Autodesk Fusion 360 part; units mm, degrees
sketch "Sketch1" plane through (0, 0, 0) normal (0, 1, 0) x (1, 0, 0)
  line L0 (2, -3.5) -> (30.5, -3.5)
  line L1 (30.5, -3.5) -> (30.5, -2)
  line L2 (30.5, -2) -> (2, -2)
  line L3 (2, -2) -> (2, -3.5)
  line L4 (12.5, -3.5) -> (20, -3.5)
  line L5 (20, -3.5) -> (20, -6.5)
  line L6 (20, -6.5) -> (12.5, -6.5)
  line L7 (12.5, -6.5) -> (12.5, -3.5)
  line L8 (12.1, -6.9) -> (20.4, -6.9)
  line L9 (20.4, -6.9) -> (20.4, -3.1)
  line L10 (20.4, -3.1) -> (12.1, -3.1)
  line L11 (12.1, -3.1) -> (12.1, -6.9)
  line L12 (0, -8.9) -> (32.5, -8.9)
  line L13 (32.5, -8.9) -> (32.5, 0)
  line L14 (32.5, 0) -> (0, 0)
  line L15 (0, 0) -> (0, -8.9)
  line L16 (30.5, -3.7) -> (26.5, -3.7)
  line L17 (26.5, -3.7) -> (26.5, -4.7)
  line L18 (26.5, -4.7) -> (30.5, -4.7)
  line L19 (30.5, -4.7) -> (30.5, -3.7)
  line L20 (26.5, -1.8) -> (30.5, -1.8)
  line L21 (30.5, -1.8) -> (30.5, -0.8)
  line L22 (30.5, -0.8) -> (26.5, -0.8)
  line L23 (26.5, -0.8) -> (26.5, -1.8)
  line L24 (2, -4.7) -> (6, -4.7)
  line L25 (6, -4.7) -> (6, -3.7)
  line L26 (6, -3.7) -> (2, -3.7)
  line L27 (2, -3.7) -> (2, -4.7)
  line L28 (2, -1.8) -> (6, -1.8)
  line L29 (6, -1.8) -> (6, -0.8)
  line L30 (6, -0.8) -> (2, -0.8)
  line L31 (2, -0.8) -> (2, -1.8)
  dimension "d1" = 28.5
  dimension "d2" = 1.5
  dimension "d3" = 7.5
  dimension "d4" = 3
  dimension "d5" = 10.5
  dimension "d6" = 0.4
  dimension "d7" = 0.4
  dimension "d8" = 0.4
  dimension "d9" = 0.4
  dimension "d10" = 2
  dimension "d11" = 2
  dimension "d12" = 2
  dimension "d13" = 2
  dimension "d30" = 4
  dimension "d31" = 1
  dimension "d32" = 0.2
  dimension "d33" = 4
  dimension "d34" = 4
  dimension "d35" = 1
  dimension "d36" = 0.2
  dimension "d37" = 4
  dimension "d38" = 4
  dimension "d39" = 1
  dimension "d40" = 4
  dimension "d41" = 1
  dimension "d42" = 4
  dimension "d43" = 4
  dimension "d44" = 0.2
  dimension "d45" = 0.2
extrude "Extrude1" add sketch "Sketch1" along normal blind 2 contours L0 L1 L2 L3 L9 L10 L11 | L12 L13 L14 L15 | L16 L17 L18 L19 | L20 L21 L22 L23 | L24 L25 L26 L27 | L28 L29 L30 L31
extrude "Extrude4" cut 1 faces at (28.4667, 2, 4) along direction (0, -1, 0) blind 1
extrude "Extrude5" add sketch "Sketch1" against normal blind 4 contours L16 L17 L18 L19 | L20 L21 L22 L23 | L24 L25 L26 L27 | L28 L29 L30 L31
sketch "Sketch3" plane through (0, 0, 4.7) normal (0, 0, 1) x (-1, 0, 0)
  line L0 (-6, 0) -> (-2, 0)
  line L1 (-2, 0) -> (-2, 4)
  line L2 (-2, 4) -> (-6, 4)
  line L3 (-6, 4) -> (-6, 0)
  circle A0 centre (-4, 2) radius 1.5
  circle A1 centre (-28.5, 2) radius 1.5
  dimension "d50" = 3
  dimension "d51" = 3
extrude "Extrude6" cut sketch "Sketch3" against normal blind 8 contours A0 | A1
equation "d5 = ( 21 / 2 ) * 1 mm"
The model under review builds one solid part; all positions refer to its coordinate system, in mm. A direction names the side the tool comes from. Give positions to 0.01 mm unless a question says otherwise; leave off trailing zeros. Order: outer loops, then holes, each group sorted by start corner. A loop starts at its lowest first (then second) coordinate and runs counter-clockwise, first axis right, second up. Notation, with made-up numbers: (-0.5, 35) - (17.5, 35) arc R9 ccw to (17.5, 46) - close; hole circle Ø2 at (75.25, 64.5). An arc over 180 degrees is marked (long way). Use CSV: the item, a comma, the result in double quotes. Start each with the question number.
Q1. We need section B-B, the plane z = 6.5. Write out the cut boundary in (x, y).
Q2. Clearance check with flat-ended pins moving along their axes: pin 1 Ø1.1 at (y, z) = (-2.5, 4) entering from -X; pin 2 Ø2.5 at (x, y) = (28.5, -2) entering from +Z; pin 3 Ø0.8 at (y, z) = (-2, 1) entering from +X; pin 4 Ø4.5 at (x, z) = (20, 5.5) entering from -Y. State where each tip first meets the part, or that it passes through.
Q3. To check wall thickness, follow line 1 along X through (y, z) = (-2, 1.45); line 2 along Y through (x, z) = (4, 1); line 3 along X through (y, z) = (0.35, 4). State the ranges of each line that lie inside material, in increasing order. Write a range as [from, to].
Q4. Tool access review of faces 5 (the flat face through (27.6, -0.6, 0.8)), 6 (the flat face through (26.5, -2, 4)), 7 (the flat face through (16.2, 0.5, 6.9)): name each direction out of +Z, -Z, +X, -X, +Y, -Y from which nothing blocks a thin tool from reaching the whole face with its end or side.
Q5. We need section A-A, the plane x = 4. Write out the cut boundary in (y, z), and give its area (3 significant figures).
Q6. We need section D-D, the plane y = -2. State how many separate pieces and enclosed holes the cut face has, and give its area (3 significant figures).
Q7. We need section C-C, the plane x = 19. Write out the cut boundary in (y, z), and give its area (3 significant figures).
Q8. The part is to be moulded in two halves that separate along Z. For faces 1 (the flat face through (20.4, 0.5, 5)), 2 (the flat face through (30, -3, 1.8)), 3 (the flat face through (16, 0.5, 8.9)), 4 (the flat face through (30.5, -2, 4)), say which applies: +Z half, -Z half, draft (parallel to the pull), parting line (faces both ways), or undercut.
Outcome:
1,outline,"(0, 0) - (12.1, 0) - (12.1, 1) - (0, 1) - close; (20.4, 0) - (32.5, 0) - (32.5, 1) - (20.4, 1) - close"
2,pin 1,"stops at x = 2"
2,pin 2,"passes through"
2,pin 3,"stops at x = 30.5"
2,pin 4,"stops at y = 0"
3,line 1,"x = [2, 2.5], [5.5, 6], [26.5, 27], [30, 30.5]"
3,line 2,"y = [-4, -3.5], [-0.5, 1]"
3,line 3,"x = [0, 12.1], [20.4, 32.5]"
4,face 5,"-Z, +X, -X, -Y"
4,face 6,"+Z, -Z, -Y"
4,face 7,"+Y, -Y"
5,outline,"(-4, 0.8) - (-3.5, 0.8) - (-3.5, 1.8) - (-4, 1.8) - close; (-4, 3.7) - (-3.5, 3.7) - (-3.5, 4.7) - (-4, 4.7) - close; (-0.5, 0.8) - (0, 0.8) - (0, 0) - (1, 0) - (1, 8.9) - (0, 8.9) - (0, 4.7) - (-0.5, 4.7) - (-0.5, 3.7) - (0, 3.7) - (0, 1.8) - (-0.5, 1.8) - close"
5,area,"10.9 mm^2"
6,separate pieces,"8"
6,enclosed holes,"0"
6,area,"4.00 mm^2"
7,outline,"(0, 0) - (1, 0) - (1, 3.1) - (0, 3.1) - close; (0, 6.9) - (1, 6.9) - (1, 8.9) - (0, 8.9) - close"
7,area,"5.10 mm^2"
8,face 1,"undercut"
8,face 2,"undercut"
8,face 3,"+Z half"
8,face 4,"draft"
